The model under review builds one solid part; all positions refer to its coordinate system, in mm. A direction names the side the tool comes from. Give positions to 0.01 mm unless a question says otherwise; leave off trailing zeros. Order: outer loops, then holes, each group sorted by start corner. A loop starts at its lowest first (then second) coordinate and runs counter-clockwise, first axis right, second up. Notation, with made-up numbers: (27.25, 0) - (69.25, 0) arc R21 ccw to (69.25, 27) - close; hole circle Ø11 at (38.25, 72). An arc over 180 degrees is marked (long way). Write item = value, one per line. Start each with the question number.
1. For P1, Ø2.5, axis at x = 3, z = -19.5, coming from the +Y side; P2, Ø2, axis at x = 2.5, z = 18.5, coming from the -Y side; P3, Ø1.5, axis at x = 2, y = 12.5, coming from the -Z side, all flat-tipped, find the tip position at first contact; note any pin that passes through.
2. We need section D-D, the plane z = 4. Give the boundary of the cut face in (x, y), and give its area (3 significant figures).
3. We need section C-C, the plane y = 3.5. Give the boundary of the cut face in (x, z).
4. We need section A-A, the plane x = 0.45. Give the boundary of the cut face in (y, z), and give its area (3 significant figures).
5. Wall thickness on probe 1 along Z at (x, y) = (2.5, -14.7); probe 2 along Z at (x, y) = (1.9, -7); probe 3 along Z at (x, y) = (3.95, 13): over which ranges is each line inside the solid? List them lowest first.
6. Machinability: for faces 1 (the flat face through (3, -2.5, -20)), 2 (the flat face through (3, 10, -16)), 3 (the flat face through (3, -14, 20)), which of the approach directions +Z, -Z, +X, -X, +Y, -Y give a long, thin tool a straight path to every point of the face, cutting with its end or side? Answer none if there is none.
7. We need section B-B, the plane z = 18.5. Give the boundary of the cut face in (x, y).
8. Mouldability with a two-part tool opening along Z and no side actions: class faces 4 (the cylindrical face through (2.971, -15.479, 17.364)), 5 (the flat face through (4, 17, 0)), 6 (the flat face through (2, 0, -21)), 7 (the flat face through (2, 10, 16)) as pulls with the +Z half, pulls with the -Z half, needs draft (parallel to the pull), parting line crosses it, or undercut.
Autodesk Inventor part; units mm, degrees
ref_plane "YZ Plane" through (0, 0, 0) normal (1, 0, 0) x (0, 1, 0)
ref_plane "XZ Plane" through (0, 0, 0) normal (0, 1, 0) x (-1, 0, 0)
ref_plane "XY Plane" through (0, 0, 0) normal (0, 0, 1) x (1, 0, 0)
sketch "Sketch1" plane through (0, 0, 0) normal (1, 0, 0) x (0, 1, 0)
  circle A0 centre (0, 0) radius 15
  line L0 (15, 15) -> (-15, 15)
  line L1 (-15, 15) -> (-15, -15) construction
  line L2 (-15, -15) -> (15, -15)
  line L3 (15, -15) -> (15, 15) construction
  line L4 (15, 15) -> (-15, -15) construction
  line L5 (-15, 15) -> (15, -15) construction
  line L6 (17, 21) -> (-17, 21)
  line L7 (-17, 21) -> (-17, -21)
  line L8 (-17, -21) -> (17, -21)
  line L9 (17, -21) -> (17, 21)
  line L10 (17, 21) -> (-17, -21) construction
  line L11 (-17, 21) -> (17, -21) construction
  circle A1 centre (13, -13) radius 1
  circle A2 centre (13, 13) radius 1
  circle A3 centre (-13, -13) radius 1
  circle A4 centre (-13, 13) radius 1
  line L12 (17, -15) -> (15, -15)
  line L13 (-15, -15) -> (-17, -15)
  line L14 (17, 15) -> (15, 15)
  line L15 (-15, 15) -> (-17, 15)
  point P0 (0, -15)
  point P1 (0, 15)
  dimension "d0" = 30
  dimension "d1" = 42
  dimension "d2" = 34
  dimension "d10" = 2
  dimension "d11" = 2
  dimension "d14" = 26
  dimension "d17" = 26
sketch "Sketch2" plane through (0, 0, 0) normal (0, 1, 0) x (-1, 0, 0)
  line L0 (190, 50) -> (-10, 50)
  line L1 (-10, 50) -> (-10, -50)
  line L2 (-10, -50) -> (190, -50)
  line L3 (190, -50) -> (190, 50)
  point P0 (0, 0)
  point P1 (-10, 0)
  dimension "d3" = 200
  dimension "d4" = 100
  dimension "d5" = 10
extrude "Extrusion1" add sketch "Sketch1" along normal blind 5 contours A0 | A0 L0 L14 L9 L12 L2 | L0 L15 L7 L6 L9 L14 | A0 L2 L13 L7 L15 L0 | L2 L12 L9 L8 L7 L13 | A1 | A2 | A3 | A4
extrude "Extrusion4" cut sketch "Sketch1" along normal blind 3 contours A0 L0 L14 L9 L12 L2 | A0 L2 L13 L7 L15 L0
extrude "Extrusion3" cut sketch "Sketch1" along normal blind 5 contours A0 | A1 | A2 | A3 | A4
sketch "Sketch3" plane through (0, -17, 21) normal (0, 0, 1) x (1, 0, 0)
  line L0 (0, 34) -> (0, 0)
  line L1 (0, 0) -> (5, 0)
  line L2 (5, 34) -> (5, 0)
  line L3 (0, 34) -> (5, 34)
  line L4 (0, 0) -> (0, 34)
  line L5 (5, 0) -> (5, 34)
  line L6 (0, 14.5) -> (5, 14.5)
  line L7 (5, 14.5) -> (5, 3)
  line L8 (5, 3) -> (0, 3)
  line L9 (0, 3) -> (0, 14.5)
  line L10 (0, 34) -> (5, 34)
  line L11 (5, 34) -> (5, 19.5)
  line L12 (5, 19.5) -> (0, 19.5)
  line L13 (0, 19.5) -> (0, 34)
  point P0 (0, 17)
  point P1 (0, 17)
  point P2 (0, 3)
  point P3 (5, 3)
  point P4 (0, 19.5)
  dimension "d26" = 3
  dimension "d27" = 5
  dimension "d29" = 2.5
extrude "Extrusion5" cut sketch "Sketch3" against normal blind 5 contours L3 L2 L12 L0 | L6 L2 L8 L0
mirror "Mirror1" about plane through (0, 0, 0) normal (0, 0, 1) of "Extrusion5"
sketch "Sketch4" plane through (0, -17, -21) normal (0, -1, 0) x (1, 0, 0)
  line L0 (5, 42) -> (5, 0)
  line L1 (0, 0) -> (5, 0)
  line L2 (0, 42) -> (5, 42)
  point P0 (0, 21)
  point P1 (2.5, 39.5)
  point P2 (2.5, 2.5)
  dimension "d39" = 2.5
  dimension "d40" = 2.5
  dimension "d41" = 2.5
  dimension "d42" = 2.5
hole "Hole1" at (2.5, -17, 18.5) at (2.5, -17, -18.5) direction (0, 1, 0) diameter 2.459 end through all
properties part number "Camera holder"
Model answer:
q1.P1 = 2.5
q1.P2 = through
q1.P3 = -16
q2.outline = (3, -17) - (5, -17) - (5, -14.46) - (3, -14.46) - close; (3, 14.46) - (5, 14.46) - (5, 17) - (3, 17) - close
q2.area = 10.2 mm2
q3.outline = (0, -16) - (5, -16) - (5, -14.59) - (3, -14.59) - (3, -15) - (0, -15) - close; (0, 15) - (3, 15) - (3, 14.59) - (5, 14.59) - (5, 16) - (0, 16) - close
q4.outline = (-17, -21) - (-14, -21) - (-14, -16) - (-2.5, -16) - (-2.5, -21) - (2.5, -21) - (2.5, -16) - (17, -16) - (17, -15) - (-17, -15) - close; (-17, 15) - (17, 15) - (17, 16) - (2.5, 16) - (2.5, 21) - (-2.5, 21) - (-2.5, 16) - (-14, 16) - (-14, 21) - (-17, 21) - close
q4.area = 148 mm2
q5.probe_1 = -21 to -19.73, -17.27 to -15, 15 to 17.27, 19.73 to 21
q5.probe_2 = -16 to -15, 15 to 16
q5.probe_3 = -16 to -14, -12 to -7.48, 7.48 to 12, 14 to 16
q6.face_1 = -Z, +X, -X
q6.face_2 = -Z, +X, -X, +Y
q6.face_3 = +Z, +X, -X
q7.outline = (0, -17) - (1.27, -17) - (1.27, -14) - (0, -14) - close; (0, -2.5) - (1.27, -2.5) - (1.27, 2.5) - (0, 2.5) - close; (3.73, -17) - (5, -17) - (5, -14) - (3.73, -14) - close; (3.73, -2.5) - (5, -2.5) - (5, 2.5) - (3.73, 2.5) - close
q8.face_4 = undercut
q8.face_5 = needs draft
q8.face_6 = pulls with the -Z half
q8.face_7 = pulls with the +Z half
